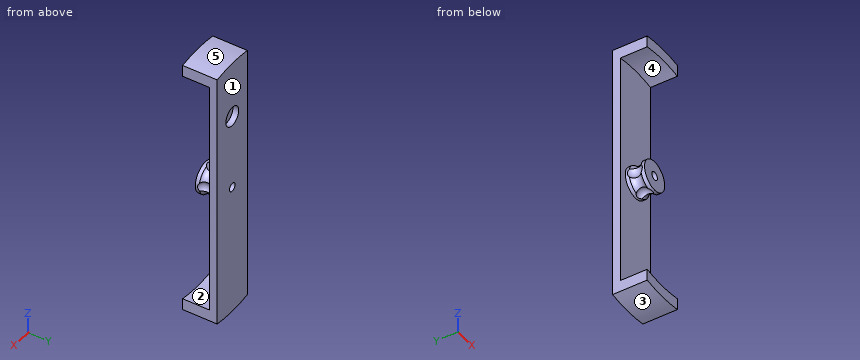
from build123d import *

# Parameters (mm, degrees)
CORTE_EXTRUS_O1_DEPTH      = 51.309044912
CORTE_EXTRUS_O1_DEPTH_BACK = 51.309044912
ESBO_O2_W                  = 96.741183006
ESBO_O2_H                  = 102.357875962
ESBO_O2_W_2                = 12
ESBO_O2_H_2                = 76.270119436
PADR_OCIRCULAR1_COUNT      = 4
ESBO_O4_R                  = 2.55
CORTE_EXTRUS_O2_DEPTH      = 1.5


with BuildPart() as part:
    # Esboço1 → Revolução1 (revolve)
    with BuildSketch(Plane.XY, mode=Mode.PRIVATE) as revolu_o1_sk:
        with BuildLine():
            Line((1.1, 7), (1.1, 0))
            Line((1.1, 0), (4, 0))
            Line((4, 0), (4, 1))
            ThreePointArc((4, 1), (3.3, 2.519868415), (4, 4.039736831))
            Line((4, 4.039736831), (4, 5))
            Line((4, 5), (32, 5))
            Line((32, 5), (32, -2))
            Line((32, -2), (35, -2))
            Line((35, -2), (35, 7))
            Line((35, 7), (3.5, 7))
            Line((3.5, 7), (1.1, 7))
        make_face()
    revolve(revolu_o1_sk.sketch.rotate(Axis((0, 0, 0), (0, 1, 0)), 90), axis=Axis((0, 0, 0), (0, 1, 0)))

    # Esboço2 → Corte-extrusão1 (cut, two sides: drawn at the far end of the back side and taken through both)
    with BuildSketch(Plane(origin=(0, 7, 0), x_dir=(1, 0, 0), z_dir=(0, 1, 0)).offset(-CORTE_EXTRUS_O1_DEPTH_BACK)):
        Rectangle(ESBO_O2_W, ESBO_O2_H)
        Rectangle(ESBO_O2_W_2, ESBO_O2_H_2, mode=Mode.SUBTRACT)
    extrude(amount=CORTE_EXTRUS_O1_DEPTH + CORTE_EXTRUS_O1_DEPTH_BACK, mode=Mode.SUBTRACT)

    # Esboço3 → Corte-Revolução1 (revolve, cut)
    with BuildSketch(Plane.XY):
        with BuildLine():
            Line((4.5, 4.519868415), (4.5, 0.519868415))
            ThreePointArc((4.5, 0.519868415), (2.5, 2.519868415), (4.5, 4.519868415))
        make_face()
    corte_revolu_o1 = revolve(axis=Axis((4.5, 4.519868415, 0), (0, -1, 0)), mode=Mode.SUBTRACT)

    # PadrãoCircular1: Corte-Revolução1 ×4 about axis
    padr_ocircular1_axis = Axis((0, 0, 0), (0, 1, 0))
    for i in range(1, PADR_OCIRCULAR1_COUNT):
        add(corte_revolu_o1.rotate(padr_ocircular1_axis, i * 360 / PADR_OCIRCULAR1_COUNT), mode=Mode.SUBTRACT)

    # Esboço4 → Corte-extrusão2 (cut)
    with BuildSketch(Plane(origin=(0, 7, 0), x_dir=(1, 0, 0), z_dir=(0, 1, 0))):
        with Locations(Location((0, -20, 0), (0, 0, 270))):
            Circle(ESBO_O4_R)
    extrude(amount=-CORTE_EXTRUS_O2_DEPTH, mode=Mode.SUBTRACT)


solid = part.part
Can you work these out from the model? Positions are in its coordinate system, mm. Face numbers are marked on the shaded views. A direction names the side the tool comes from. Give positions to 0.01 mm unless a question says otherwise; leave off trailing zeros. Write each loop counter-clockwise with the first axis right and the second up, starting at its lowest first coordinate (ties: lowest second). Pieces come first, ordered by that corner, then holes. Notation, with made-up numbers: (79.5, 46) -> (121.5, 46) arc R22 ccw to (121.5, 61) -> close; hole circle Ø5 at (-32, 35). An arc over 180 degrees is marked (long way). Answer as a JSON object with one key per item and string values. Group by question number.
Item 1: We'd pull the mould along Z, two halves only. Please class the marked faces 3, 4 and 5: +Z half, -Z half, draft (parallel to the pull), parting line (faces both ways), or undercut.
Item 2: Please list where these lines run through material, in increasing order: line 1 (X direction, y = 6.3, z = 20); line 2 (Z direction, x = 2.5, y = 0.5); line 3 (Z direction, x = -4, y = 1.25). Write a range as [from, to].
Item 3: Suppose I cut it at B-B (z = 0). Please give me the cut outline in (x, y), plus the area to 3 significant figures.
Item 4: For the marked faces 1 and 2, which set-ups out of +Z, -Z, +X, -X, +Y, -Y let a thin tool reach every point of the face, with its end or its side?
Item 5: Suppose I cut it at C-C (y = 1.75). Please give me the cut outline in (x, z).
Item 6: I'm going to push flat-ended pins straight in: P1, Ø6, axis at x = -3, z = -5, coming from the -Y side; P2, Ø5, axis at x = -4.5, y = 4, coming from the -Z side; P3, Ø6.5, axis at x = 0, z = 20, coming from the -Y side; P4, Ø4, axis at y = 2.5, z = 24.5, coming from the -X side. Where does each tip first touch, or does it pass through?
Item 7: Suppose I cut it at D-D (z = 20). Please give me the cut outline in (x, y), plus the area to 4 significant figures.
Item 8: Suppose I cut it at A-A (x = 0). Please give me the cut outline in (y, z), plus the area to 3 significant figures.
Findings:
{
 "1": {"face 3": "-Z half", "face 4": "undercut", "face 5": "+Z half"},
 "2": {"line 1": "x = [-6, -2.55], [2.55, 6]", "line 2": "z = [-34.91, -31.9], [-3.12, 3.12], [31.9, 34.91]", "line 3": "z = [-34.77, -31.75], [31.75, 34.77]"},
 "3": {"outline": "(-6, 5) -> (-4, 5) -> (-4, 4.46) arc R2 cw to (-4, 0.58) -> (-4, 0) -> (-1.1, 0) -> (-1.1, 7) -> (-6, 7) -> close; (1.1, 0) -> (4, 0) -> (4, 0.58) arc R2 cw to (4, 4.46) -> (4, 5) -> (6, 5) -> (6, 7) -> (1.1, 7) -> close", "area": "40.0 mm²"},
 "4": {"face 1": "+Z, -Z, +X, -X, +Y", "face 2": "-Y"},
 "5": {"outline": "(-6, -34.48) arc R35 ccw to (6, -34.48) -> (6, -31.43) arc R32 cw to (-6, -31.43) -> close; (-6, 31.43) arc R32 cw to (6, 31.43) -> (6, 34.48) arc R35 ccw to (-6, 34.48) -> close; (-3.2, -1.31) arc R3.45 ccw to (-1.31, -3.2) arc R1.85 cw to (1.31, -3.2) arc R3.45 ccw to (3.2, -1.31) arc R1.85 cw to (3.2, 1.31) arc R3.45 ccw to (1.31, 3.2) arc R1.85 cw to (-1.31, 3.2) arc R3.45 ccw to (-3.2, 1.31) arc R1.85 cw to start; hole circle Ø2.2 at (0, 0)"},
 "6": {"P1": "stops at y = 0", "P2": "stops at z = -34.94", "P3": "stops at y = 5", "P4": "passes through"},
 "7": {"outline": "(-6, 5) -> (6, 5) -> (6, 7) -> (2.55, 7) -> (2.55, 5.5) -> (-2.55, 5.5) -> (-2.55, 7) -> (-6, 7) -> close", "area": "16.35 mm²"},
 "8": {"outline": "(-2, -35) -> (7, -35) -> (7, -1.1) -> (0, -1.1) -> (0, -4) -> (0.58, -4) arc R2 cw to (4.46, -4) -> (5, -4) -> (5, -32) -> (-2, -32) -> close; (-2, 32) -> (5, 32) -> (5, 4) -> (4.46, 4) arc R2 cw to (0.58, 4) -> (0, 4) -> (0, 1.1) -> (7, 1.1) -> (7, 17.45) -> (5.5, 17.45) -> (5.5, 22.55) -> (7, 22.55) -> (7, 35) -> (-2, 35) -> close", "area": "190 mm²"}
}
